```python
from build123d import *

# Parameters (mm, degrees)
SKETCH1_R           = 10
BOSS_EXTRUDE1_DEPTH = 172.5
SKETCH4_R           = 7.5
BOSS_EXTRUDE2_DEPTH = 40
SKETCH5_R           = 6
BOSS_EXTRUDE3_DEPTH = 12
CHAMFER1_SIZE       = 0.5


with BuildPart() as part:
    # Sketch1 → Boss-Extrude1 (new, symmetric)
    with BuildSketch(Plane.XY):
        Circle(SKETCH1_R)
    extrude(amount=BOSS_EXTRUDE1_DEPTH, both=True)

    # Sketch4 → Boss-Extrude2 (add)
    with BuildSketch(Plane.XY.offset(172.5)):
        Circle(SKETCH4_R)
    extrude(amount=BOSS_EXTRUDE2_DEPTH)

    # Sketch5 → Boss-Extrude3 (add)
    with BuildSketch(Plane.XY.offset(212.5)):
        Circle(SKETCH5_R)
    extrude(amount=BOSS_EXTRUDE3_DEPTH)

    # Chamfer1
    chamfer1_edges = [part.edges().sort_by_distance(p)[0] for p in [
        (-6, 0, 224.5),
        (-10, 0, -172.5),
        (-10, 0, 172.5),
        (-7.5, 0, 212.5),
    ]]
    chamfer(chamfer1_edges, length=CHAMFER1_SIZE)


solid = part.part
```
The model under review builds one solid part; all positions refer to its coordinate system, in mm. A direction names the side the tool comes from. Round coordinates to 2 decimals unless told otherwise and drop trailing zeros. Write each loop counter-clockwise with the first axis right and the second up, starting at its lowest first coordinate (ties: lowest second). Pieces come first, ordered by that corner, then holes.
(1) We need section C-C on z = -89. Give the boundary of the cut face in (x, y).
(2) Insertion check: pin 1 (3 mm diameter, centred on x = 3, y = 6.5, fed in from +Z); pin 2 (1 mm diameter, centred on x = -4, z = 133.5, fed in from +Y); pin 3 (4 mm diameter, centred on y = -5.5, z = 171, fed in from +X). Each pin has a flat end and moves straight along its axis. Give the tip position at first contact, or say it passes through.
(3) Machinability: for faces 1 (the cylindrical face through (-6, 0, 218)), 2 (the flat face through (0, 0, -172.5)), which of the approach directions +Z, -Z, +X, -X, +Y, -Y give a long, thin tool a straight path to every point of the face, cutting with its end or side? Answer none if there is none.
(4) Wall thickness on L1, parallel to X at y = 0.75, z = 167; L2, parallel to Z at x = 5.5, y = 5.25; L3, parallel to Y at x = -1.25, z = -87: over which ranges is each line inside the solid? List them lowest first.
(5) We need section A-A on y = 0. Give the boundary of the cut face in (x, z), and give its area (3 significant figures).
Findings below:
1. outline: circle Ø20 at (0, 0)
2. pin 1: stops at z = 224.34
2. pin 2: stops at y = 9.37
2. pin 3: stops at x = 9.37
3. face 1: +Z
3. face 2: -Z, +X, -X, +Y, -Y
4. L1: x = -9.97 to 9.97
4. L2: z = -172.5 to 172.5
4. L3: y = -9.92 to 9.92
5. outline: (-10, -172) - (-9.5, -172.5) - (9.5, -172.5) - (10, -172) - (10, 172) - (9.5, 172.5) - (7.5, 172.5) - (7.5, 212) - (7, 212.5) - (6, 212.5) - (6, 224) - (5.5, 224.5) - (-5.5, 224.5) - (-6, 224) - (-6, 212.5) - (-7, 212.5) - (-7.5, 212) - (-7.5, 172.5) - (-9.5, 172.5) - (-10, 172) - close
5. area: 7,640 mm2
